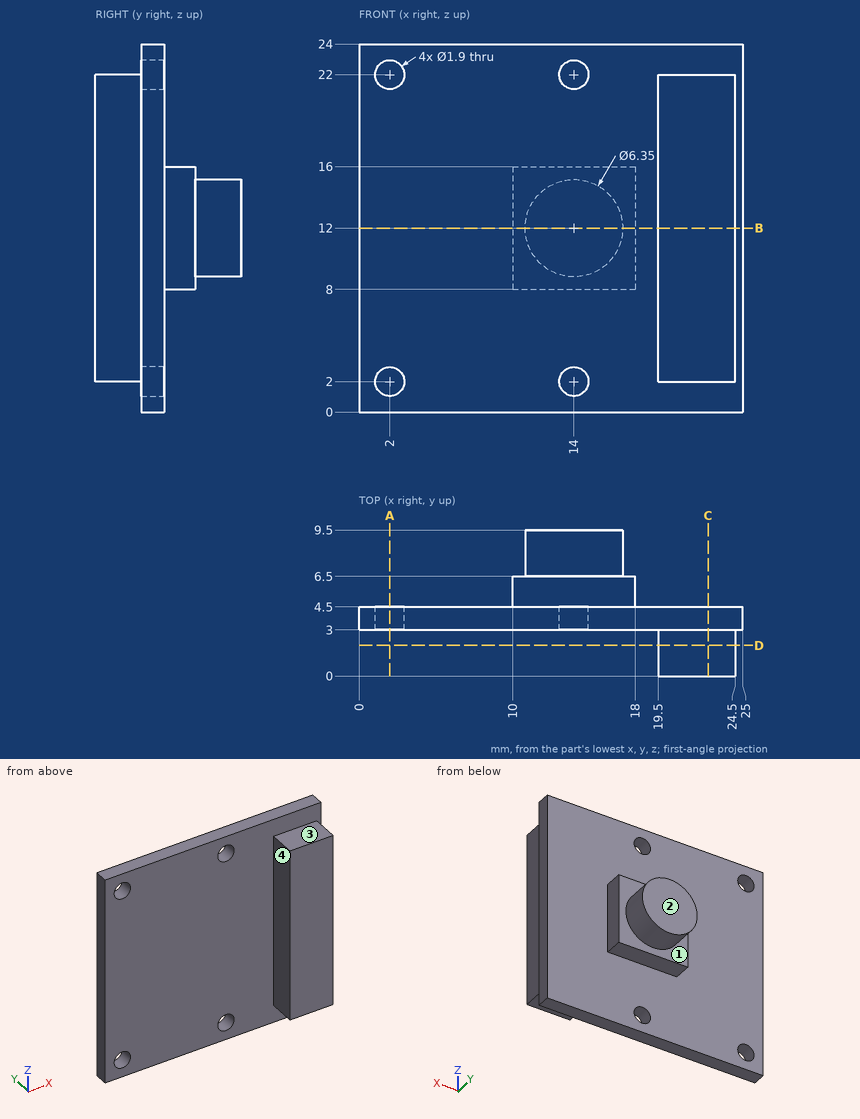
Geometry: see drawing. Coordinates: mm, zero at the bounding-box minimum. A direction names the side the tool comes from. Coordinates: 2 decimals unless noted, no trailing zeros. Loops run counter-clockwise (first coordinate to the right, second up) from the corner with the lowest first, then second, coordinate; pieces in that order, holes last. Notation, with made-up numbers: (4, 20.5) -> (44, 20.5) arc R19 ccw to (44, 38.5) -> close; hole circle Ø6 at (76.5, -3.75). An arc over 180 degrees is marked (long way). Write item = value, one per line. Start each with the question number.
Item 1: Cut plane B-B, the plane z = 12. Return loops of the section in (x, y) (3 decimals).
Item 2: First-contact query: P1, Ø1, axis at y = 6, z = 13.5, coming from the -X side; P2, Ø2, axis at y = 6, z = 11.5, coming from the +X side; P3, Ø2, axis at x = 14, z = 22, coming from the -Y side. Flat tips, straight axial feed; report the tip coordinate or a pass-through.
Item 3: Cut plane C-C, the plane x = 22.75. Return loops of the section in (y, z), plus the area to 3 significant figures.
Item 4: Reachability of the marked faces 1, 2, 3 and 4 from +Z, -Z, +X, -X, +Y, -Y: full face, straight path, thin tool, end or side. Return the list, or none.
Item 5: Material intervals for line 1 (X direction, y = 3.55, z = 22); line 2 (Y direction, x = 17.25, z = 22); line 3 (Y direction, x = 15, z = 15.25), sorted ascending.
Item 6: Cut plane A-A, the plane x = 2. Return loops of the section in (y, z).
Item 7: Cut plane D-D, the plane y = 2. Return loops of the section in (x, z).
Ans:
q1.outline = (0, 3) -> (19.5, 3) -> (19.5, 0) -> (24.5, 0) -> (24.5, 3) -> (25, 3) -> (25, 4.5) -> (18, 4.5) -> (18, 6.5) -> (17.175, 6.5) -> (17.175, 9.5) -> (10.825, 9.5) -> (10.825, 6.5) -> (10, 6.5) -> (10, 4.5) -> (0, 4.5) -> close
q2.P1 = 10
q2.P2 = 18
q2.P3 = 3
q3.outline = (0, 2) -> (3, 2) -> (3, 0) -> (4.5, 0) -> (4.5, 24) -> (3, 24) -> (3, 22) -> (0, 22) -> close
q3.area = 96.0 mm²
q4.face_1 = +Y
q4.face_2 = +Z, -Z, +X, -X, +Y
q4.face_3 = +Z, +X, -X, -Y
q4.face_4 = +Z, -Z, -X, -Y
q5.line_1 = 0 to 1.05, 2.95 to 13.05, 14.95 to 25
q5.line_2 = 3 to 4.5
q5.line_3 = 3 to 6.5
q6.outline = (3, 0) -> (4.5, 0) -> (4.5, 1.05) -> (3, 1.05) -> close; (3, 2.95) -> (4.5, 2.95) -> (4.5, 21.05) -> (3, 21.05) -> close; (3, 22.95) -> (4.5, 22.95) -> (4.5, 24) -> (3, 24) -> close
q7.outline = (19.5, 2) -> (24.5, 2) -> (24.5, 22) -> (19.5, 22) -> close
